```python
from build123d import *

# Parameters (mm, degrees)
F0_R     = 26.697036
F0_R_2   = 16.515215
F1_DEPTH = 146.796286
F3_DEPTH = 146.796286


with BuildPart() as f1:
    # F0 (on Top) → F1 (new body)
    with BuildSketch(Plane.XY):
        Circle(F0_R)
        Circle(F0_R_2, mode=Mode.SUBTRACT)
    extrude(amount=F1_DEPTH)

    # F2 (on face) → F3 (cut, through all)
    with BuildSketch(Plane(origin=(0, 0, 0), x_dir=(1, 0, 0), z_dir=(0, 0, -1))):
        with BuildLine():
            Line((-8.89, -20.32), (8.89, -20.32))
            Line((8.89, -20.32), (8.89, -13.918341))
            ThreePointArc((8.89, -13.918341), (0, -16.515215), (-8.89, -13.918341))
            Line((-8.89, -13.918341), (-8.89, -20.32))
        make_face()
    extrude(amount=-F3_DEPTH, mode=Mode.SUBTRACT)


solid = f1.part
```
Work out the finished part from the listing and answer in its coordinate system (mm). A direction names the side the tool comes from. Give positions to 0.01 mm unless a question says otherwise; leave off trailing zeros. Write each loop counter-clockwise with the first axis right and the second up, starting at its lowest first coordinate (ties: lowest second). Pieces come first, ordered by that corner, then holes.
(1) The part is cut by section B-B on y = 0. Write down the section's boundary in (x, z).
Final values:
outline: (-26.7, 0) - (-16.52, 0) - (-16.52, 146.8) - (-26.7, 146.8) - close; (16.52, 0) - (26.7, 0) - (26.7, 146.8) - (16.52, 146.8) - close
(2) The part is cut by section A-A on x = 0. Write down the section's boundary in (y, z), plus the area to 3 significant figures.
Final values:
outline: (-26.7, 0) - (-16.52, 0) - (-16.52, 146.8) - (-26.7, 146.8) - close; (20.32, 0) - (26.7, 0) - (26.7, 146.8) - (20.32, 146.8) - close
area: 2,430 mm2
(3) The part is cut by section C-C on z = 42.5. Write down the section's boundary in (x, y).
Final values:
outline: circle Ø53.39 at (0, 0); hole (-8.89, 13.92) arc R16.52 ccw (long way) to (8.89, 13.92) - (8.89, 20.32) - (-8.89, 20.32) - close
(4) Straight lines are drawn through the part: line 1 (Y direction, x = 12, z = 78.5); line 2 (Y direction, x = 5.5, z = 25); line 3 (Y direction, x = 17, z = 133). For each, find the intervals that lie inside material, in ascending order.
Final values:
line 1: y = -23.85 to -11.35, 11.35 to 23.85
line 2: y = -26.12 to -15.57, 20.32 to 26.12
line 3: y = -20.58 to 20.58
(5) Flat-ended cylindrical pins translate along their axes: pin 1 Ø3 at (y, z) = (18.5, 45) entering from +X; pin 2 Ø19.5 at (x, z) = (-4.5, 109.5) entering from -Y; pin 3 Ø3 at (x, z) = (6.5, 64.5) entering from -Y. Find the tip coordinate at first contact, or state that the pin passes through.
Final values:
pin 1: stops at x = 20.58
pin 2: stops at y = -26.7
pin 3: stops at y = -26.22
(6) The part is cut by section D-D on y = -22.5. Write down the section's boundary in (x, z), plus the area to 3 significant figures.
Final values:
outline: (-14.37, 0) - (14.37, 0) - (14.37, 146.8) - (-14.37, 146.8) - close
area: 4,220 mm2
(7) Which of the six approach directions +Z, -Z, +X, -X, +Y, -Y give full straight-line access (tool end or side, diameter ignored) to faces 4 (the flat face through (8.89, 17, 72)), 5 (the flat face through (0, -17, 146.796))?
Final values:
face 4: +Z, -Z
face 5: +Z, +X, -X, +Y, -Y
(8) The mould has two halves that part along Y. Classify faces 1 (the flat face through (-8.89, 17, 72)), 2 (the flat face through (0, -17, 0)), 3 (the cylindrical face through (-21.19, -16.24, 72.37)): pulls with the +Y half, pulls with the -Y half, needs draft (parallel to the pull), parting line crosses it, or undercut.
Final values:
face 1: undercut
face 2: needs draft
face 3: parting line crosses it
